Autodesk Inventor part; units mm, degrees
ref_plane "YZ Plane" through (0, 0, 0) normal (1, 0, 0) x (0, 1, 0)
ref_plane "XZ Plane" through (0, 0, 0) normal (0, 1, 0) x (-1, 0, 0)
ref_plane "XY Plane" through (0, 0, 0) normal (0, 0, 1) x (1, 0, 0)
sketch "Esquisse1" plane through (0, 0, 0) normal (0, 0, 1) x (1, 0, 0)
  line L0 (0, 0) -> (-27.546, -25.0426) construction
  line L1 (0, 0) -> (23.0277, -27.4577) construction
  circle A0 centre (-18.0975, -16.4528) radius 1.25
  circle A1 centre (15.7127, -18.7355) radius 1.25
  arc A2 (-16.6894, -17.8731) -> (14.1299, -19.9581) centre (0, 0) ccw
  arc A3 (-16.6894, -17.8731) -> (-19.3824, -14.9201) centre (-18.0975, -16.4528) ccw
  arc A4 (17.0433, -17.2424) -> (14.1299, -19.9581) centre (15.7127, -18.7355) ccw
  line L2 (0, 0) -> (-29.5508, 10.7556) construction
  line L3 (-17.8311, 0) -> (17.1748, 0) construction
  line L4 (0, 2.0526) -> (0, -2.2236) construction
  arc A5 (-25.923, -2) -> (25.923, -2) centre (0, 0) ccw
  circle A6 centre (0, 0) radius 22.5 construction
  arc A7 (-16.6894, -17.8731) -> (14.1299, -19.9581) centre (0, 0) ccw
  arc A8 (-16.6894, -17.8731) -> (14.1299, -19.9581) centre (0, 0) ccw
  circle A9 centre (-25.3169, 1.1605) radius 1.25
  circle A10 centre (25.3169, 1.1605) radius 1.25
  line L5 (24.0891, 2.7784) -> (24.0891, 12.8348)
  line L6 (25.8363, 12.8348) -> (24.0891, 12.8348)
  line L7 (-25.923, 6.143) -> (-25.923, 12.7847)
  line L8 (-24.2942, 2.9148) -> (-24.2942, 12.7847)
  line L9 (-24.2942, 12.7847) -> (-25.923, 12.7847)
  arc A11 (-24.4506, -0.676) -> (-19.3824, -14.9201) centre (0, 0) ccw
  arc A12 (-24.4506, -0.676) -> (-19.3824, -14.9201) centre (0, 0) ccw
  arc A13 (-24.4506, -0.676) -> (-24.2942, 2.9148) centre (-25.3169, 1.1605) ccw
  arc A14 (17.0433, -17.2424) -> (24.2376, -0.5599) centre (0, 0) ccw
  arc A15 (17.0433, -17.2424) -> (24.2376, -0.5599) centre (0, 0) ccw
  arc A16 (17.0433, -17.2424) -> (24.2376, -0.5599) centre (0, 0) ccw
  arc A17 (24.0891, 2.7784) -> (24.2376, -0.5599) centre (25.3169, 1.1605) ccw
  line L10 (25.8363, 3.0919) -> (25.8363, 3.124)
  line L11 (25.8363, 6.3239) -> (25.8363, 12.8348)
  line L12 (25.8363, 6.3239) -> (25.9915, 6)
  line L13 (-36, 4) -> (-26.9495, 4)
  line L14 (-36, 6) -> (-26, 6)
  line L15 (-36, 4) -> (-36, 6)
  line L16 (-26, 6) -> (-25.9915, 6)
  line L17 (-25.9915, 6) -> (-25.923, 6.143)
  line L18 (-26.9495, 4) -> (-26.9495, 2.3678)
  line L19 (-25.923, -2) -> (-26.9495, -0.0468)
  arc A18 (-26.9495, 2.3678) -> (-26.9495, -0.0468) centre (-25.3169, 1.1605) ccw
  arc A19 (-24.4506, -0.676) -> (-24.2942, 2.9148) centre (-25.3169, 1.1605) ccw
  line L20 (25.9915, 6) -> (25.923, 6.143)
  line L21 (36, 4) -> (26.9495, 4)
  line L22 (36, 6) -> (26, 6)
  line L23 (36, 4) -> (36, 6)
  line L24 (26.9495, 4) -> (26.9495, 2.3678)
  line L25 (25.923, -2) -> (26.9495, -0.0468)
  arc A20 (26.9495, -0.0468) -> (26.9495, 2.3678) centre (25.3169, 1.1605) ccw
  line L26 (25.9915, 6) -> (26, 6)
  point P0 (29.8237, -2)
  point P1 (-36, -2)
  point P2 (-26.3114, 9.5766)
  dimension "d35" = 2.5
  dimension "d36" = 2.5
  dimension "d37" = 4
  dimension "d38" = 4
  dimension "d39" = 20
  dimension "d52" = 45
  dimension "d65" = 2.5
  dimension "d81" = 10
ref_plane "Plan de construction1" through (-42, 0, 0) normal (0, 1, 0) x (1, 0, 0)
ref_plane "Plan de construction2" through (-36, 0, 0) normal (0, 1, 0) x (1, 0, 0)
sketch "Esquisse3" plane through (-36, 0, 0) normal (0, 1, 0) x (1, 0, 0)
  line L0 (0, 0) -> (10, 0)
  line L1 (0, 0) -> (0, -8)
  line L2 (10, -8) -> (0, -8)
  line L3 (10, 0) -> (10, -8)
  circle A0 centre (4, -4) radius 2.15
  line L4 (62, 0) -> (72, 0)
  line L5 (62, 0) -> (62, -8)
  line L6 (72, -8) -> (62, -8)
  line L7 (72, 0) -> (72, -8)
  circle A1 centre (68, -4) radius 2.15
  point P0 (36, 0)
  dimension "d48" = 4.3
  dimension "d73" = 4
  dimension "d74" = 4.3
  dimension "d75" = 4
extrude "Extrusion16" add sketch "Esquisse1" along normal blind 8
extrude "Extrusion17" cut sketch "Esquisse3" along normal blind 8 contours A0 | A1
properties part number "anneau2"
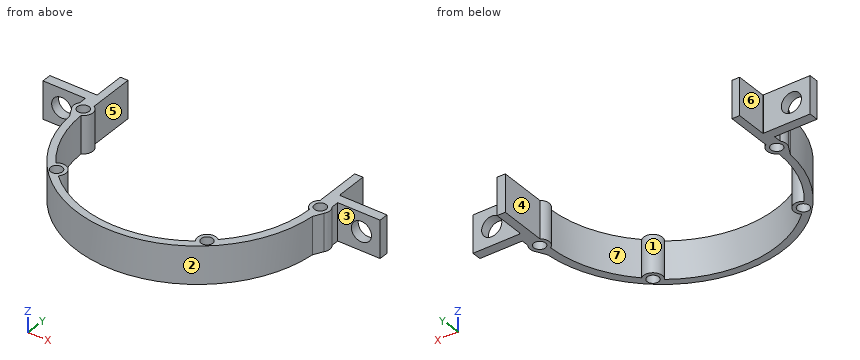
Source: CAD feature listing. Evaluate the final solid. Frame: model axes, mm. Face numbers are marked on the shaded views. A direction names the side the tool comes from. Coordinates: 2 decimals unless noted, no trailing zeros. Write each loop counter-clockwise with the first axis right and the second up, starting at its lowest first coordinate (ties: lowest second). Pieces come first, ordered by that corner, then holes. Notation, with made-up numbers: (22.25, 72.25) - (61.25, 72.25) arc R17 ccw to (61.25, 96.25) - close; hole circle Ø3 at (-9.75, -18). An arc over 180 degrees is marked (long way). Answer as a JSON object with one key per item and string values.
Q1. Section query C-C, the plane z = 1. State how many separate pieces and enclosed holes the cut face has, plus the area to 3 significant figures.
Ans:
{"separate pieces": "1", "enclosed holes": "4", "area": "219 mm2"}
Q2. Section query A-A, the plane x = -32. Output: boundary loops of the cut face in (y, z).
Ans:
{"outline": "(4, 0) - (6, 0) - (6, 1.85) - (4, 1.85) - close; (4, 6.15) - (6, 6.15) - (6, 8) - (4, 8) - close"}
Q3. Draft query along X for the marked faces 1, 2, 3 and 4. Return one class per face: released by +X, released by -X, zero draft, split by the parting line, or undercut.
Ans:
{"face 1": "undercut", "face 2": "split by the parting line", "face 3": "zero draft", "face 4": "undercut"}
Q4. Section query B-B, the plane y = -22.5. Output: boundary loops of the cut face in (x, z).
Ans:
{"outline": "(-13.03, 0) - (-9.58, 0) - (-9.58, 8) - (-13.03, 8) - close; (9.58, 0) - (13.03, 0) - (13.03, 8) - (9.58, 8) - close"}
Q5. Set-up query: the marked faces 5, 6 and 7. Return all of +Z, -Z, +X, -X, +Y, -Y with unobstructed straight access to the full face (end or side cutting, diameter ignored); none if empty.
Ans:
{"face 5": "+Z, -Z, +Y", "face 6": "+Z, -Z, -X, +Y", "face 7": "+Z, -Z"}
Q6. First-contact query: pin 1 Ø2.5 at (x, z) = (-32, 5) entering from -Y; pin 2 Ø1.8 at (y, z) = (3, 3.5) entering from -X; pin 3 Ø2.5 at (x, z) = (-29, 4.5) entering from +Y. Flat tips, straight axial feed; report the tip coordinate or a pass-through.
Ans:
{"pin 1": "stops at y = 4", "pin 2": "stops at x = -27.12", "pin 3": "stops at y = 6"}
Q7. Material intervals for line 1 (Z direction, x = -32, y = 4.65); line 2 (X direction, y = -16.5, z = 2.25); line 3 (X direction, y = -4, z = 3), sorted ascending. Write a range as [from, to].
Ans:
{"line 1": "z = [0, 1.85], [6.15, 8]", "line 2": "x = [-20.09, -19.35], [-16.85, -16.1], [17.76, 20.09]", "line 3": "x = [-25.69, -24.13], [23.91, 25.69]"}
